Read the model definition and answer for the solid it produces. Units are mm, in the model's axes. A direction names the side the tool comes from. Coordinates: 2 decimals unless noted, no trailing zeros. Order: outer loops, then holes, each group sorted by start corner. A loop starts at its lowest first (then second) coordinate and runs counter-clockwise, first axis right, second up. Notation, with made-up numbers: (15, 17.25) -> (73, 17.25) arc R23 ccw to (73, 47.25) -> close; hole circle Ø3 at (56, 22). An arc over 180 degrees is marked (long way). Answer in a Markdown table with one row per item.
from build123d import *

# Parameters (mm, degrees)
CROQUIS2_W              = 40
CROQUIS2_H              = 40
SALIENTE_EXTRUIR1_DEPTH = 2.5
CROQUIS3_R              = 2
CORTAR_EXTRUIR1_DEPTH   = 2.5
CORTAR_EXTRUIR2_DEPTH   = 16.5
CROQUIS7_W              = 0.5
CROQUIS7_H              = 3
SALIENTE_EXTRUIR2_DEPTH = 4


with BuildPart() as part:
    # Croquis1 → Revolución1 (revolve)
    with BuildSketch(Plane.XY, mode=Mode.PRIVATE) as revoluci_n1_sk:
        Polygon((0, 0), (-93.552786405, 0), (-98.552786405, 0), (-98.552786405, 1), (-96.552786405, 1), (-96.552786405, 4), (-93.552786405, 4), (-93.552786405, 15), (-54.552786405, 15), (-54.552786405, 14), (-54.052786405, 14), (-54.052786405, 15), (-32.052786405, 15), (-32.052786405, 9.5), (-20.052786405, 9.5), (-20.052786405, 3), (0, 3), align=None)
    revolve(revoluci_n1_sk.sketch.rotate(Axis((0, 0, 0), (-1, 0, 0)), 90), axis=Axis((0, 0, 0), (-1, 0, 0)))

    # Croquis2 → Saliente-Extruir1 (add)
    with BuildSketch(Plane(origin=(-32.052786405, 0, 0), x_dir=(0, 0, -1), z_dir=(1, 0, 0))):
        Rectangle(CROQUIS2_W, CROQUIS2_H)
    extrude(amount=-SALIENTE_EXTRUIR1_DEPTH)

    # Croquis3 → Cortar-Extruir1 (cut)
    with BuildSketch(Plane(origin=(-32.052786405, 0, 0), x_dir=(0, 0, -1), z_dir=(1, 0, 0))):
        with Locations((-15, 15)):
            Circle(CROQUIS3_R)
        with Locations((15, 15)):
            Circle(CROQUIS3_R)
        with Locations((-15, -15)):
            Circle(CROQUIS3_R)
        with Locations((15, -15)):
            Circle(CROQUIS3_R)
    extrude(amount=-CORTAR_EXTRUIR1_DEPTH, mode=Mode.SUBTRACT)

    # Croquis6 → Cortar-Extruir2 (cut)
    with BuildSketch(Plane(origin=(0, 0, 0), x_dir=(0, 0, -1), z_dir=(1, 0, 0))):
        with BuildLine():
            Line((-1.8, 2.4), (0, 2.4))
            Line((0, 2.4), (1.8, 2.4))
            ThreePointArc((1.8, 2.4), (0, 3), (-1.8, 2.4))
        make_face()
    extrude(amount=-CORTAR_EXTRUIR2_DEPTH, mode=Mode.SUBTRACT)

    # Croquis7 → Saliente-Extruir2 (add)
    with BuildSketch(Plane.ZY.offset(93.552786405)):
        with Locations((-10, 0)):
            Rectangle(CROQUIS7_W, CROQUIS7_H)
        with Locations((10, 0)):
            Rectangle(CROQUIS7_W, CROQUIS7_H)
    extrude(amount=SALIENTE_EXTRUIR2_DEPTH)


solid = part.part
Q1. Consider line 1 (Y direction, x = -33.1, z = 15); line 2 (X direction, y = 16.5, z = -11); line 3 (X direction, y = -3, z = -8). Determine where each line is inside the solid, lowest interval first.
Outcome:
| item | result |
|---|---|
| line 1 | -20 to -17, -13 to 13, 17 to 20 |
| line 2 | -34.55 to -32.05 |
| line 3 | -93.55 to -20.05 |
Q2. For faces 1 (the face through (-10, -3, 0)), 2 (the face through (-95.032, 3.905, 0.867)), 3 (the face through (-96, 0, -9.75)), 4 (the face through (-96, 0, 10.25)), determine the directions among +Z, -Z, +X, -X, +Y, -Y from which every point of the face is accessible in a straight line to the end or side of a thin tool.
Outcome:
| item | result |
|---|---|
| face 1 | +X |
| face 2 | -X |
| face 3 | -X, +Y, -Y |
| face 4 | +Z, -X, +Y, -Y |
Q3. The part is cut by section C-C (x = -70.5). Write down the section's boundary in (y, z), then the cut area to 3 significant figures.
Outcome:
| item | result |
|---|---|
| outline | circle Ø30 at (0, 0) |
| area | 707 mm² |
Q4. The part is cut by section B-B (x = -18.5). Write down the section's boundary in (y, z), then the cut area to 3 significant figures.
Outcome:
| item | result |
|---|---|
| outline | circle Ø6 at (0, 0) |
| area | 28.3 mm² |
Q5. Given pin 1 (5 mm diameter, centred on x = -75, z = 1.5, fed in from -Y); pin 2 (1 mm diameter, centred on y = -9.5, z = 3, fed in from -X); pin 3 (1.5 mm diameter, centred on x = -30, y = -6, fed in from +Z); pin 4 (3.5 mm diameter, centred on y = 15, z = 15, fed in from +X), each flat-ended and moving along its own axis, determine where each tip first touches the part or whether it passes through.
Outcome:
| item | result |
|---|---|
| pin 1 | y = -15 |
| pin 2 | x = -93.55 |
| pin 3 | z = 7.92 |
| pin 4 | through |
